Work out the finished part from the listing and answer in its coordinate system (mm). A direction names the side the tool comes from. Coordinates: 2 decimals unless noted, no trailing zeros. Order: outer loops, then holes, each group sorted by start corner. A loop starts at its lowest first (then second) coordinate and runs counter-clockwise, first axis right, second up. Notation, with made-up numbers: M 81,-30 L 137,-30 A17 cw 137,-20 Z; hole C -36.5,7 d2. An arc over 180 degrees is marked long. Use a Markdown table: item, result.
from build123d import *

# Parameters (mm, degrees)
SKETCH1_R           = 2.413
BOSS_EXTRUDE1_DEPTH = 45.212
SKETCH1_4_W         = 3.937
SKETCH1_4_H         = 2.794
BOSS_EXTRUDE2_DEPTH = 26.162
CUT_EXTRUDE1_START  = -24.892
SKETCH2_W           = 15.24
SKETCH2_H           = 11.43
SKETCH2_R           = 2.413
CUT_EXTRUDE1_DEPTH  = 24.892


with BuildPart() as part:
    # Sketch1 → Boss-Extrude1 (new body)
    with BuildSketch(Plane(origin=(0, 0, 0), x_dir=(1, 0, 0), z_dir=(0, 1, 0))):
        Polygon((40.25170153, 21.085507102), (40.25170153, 37.214507102), (21.20170153, 37.214507102), (21.20170153, 34.674507102), (8.50170153, 34.674507102), (8.50170153, 30.864507102), (21.20170153, 30.864507102), (21.20170153, 5.718507102), (8.50170153, 5.718507102), (8.50170153, 1.908507102), (21.20170153, 1.908507102), (21.20170153, -0.631492898), (40.25170153, -0.631492898), (40.25170153, 15.497507102), (32.37770153, 15.497507102), (32.37770153, 21.085507102), align=None)
        with Locations(Location((32.37770153, 5.591507102, 0), (0, 0, 90))):
            Circle(SKETCH1_R, mode=Mode.SUBTRACT)
        with Locations(Location((32.37770153, 30.991507102, 0), (0, 0, 90))):
            Circle(SKETCH1_R, mode=Mode.SUBTRACT)
    extrude(amount=BOSS_EXTRUDE1_DEPTH)

    # Sketch1_4 → Boss-Extrude2 (add)
    with BuildSketch(Plane(origin=(0, 0, 0), x_dir=(1, 0, 0), z_dir=(0, 1, 0))):
        with Locations((38.28320153, 19.688507102)):
            Rectangle(SKETCH1_4_W, SKETCH1_4_H)
        with Locations((34.34620153, 19.688507102)):
            Rectangle(SKETCH1_4_W, SKETCH1_4_H)
        with Locations((34.34620153, 16.894507102)):
            Rectangle(SKETCH1_4_W, SKETCH1_4_H)
        with Locations((38.28320153, 16.894507102)):
            Rectangle(SKETCH1_4_W, SKETCH1_4_H)
    extrude(amount=BOSS_EXTRUDE2_DEPTH)

    # Sketch2 → Cut-Extrude1 (cut)
    # profile 1 of 2: a face of its own
    with BuildSketch(Plane(origin=(0, 45.212, 0), x_dir=(1, 0, 0), z_dir=(0, 1, 0)).offset(CUT_EXTRUDE1_START)):
        with Locations((32.63170153, 5.083507102)):
            Rectangle(SKETCH2_W, SKETCH2_H)
        with Locations(Location((32.37770153, 5.591507102, 0), (0, 0, 90))):
            Circle(SKETCH2_R, mode=Mode.SUBTRACT)
    # profile 2 of 2: a face of its own
    with BuildSketch(Plane(origin=(0, 45.212, 0), x_dir=(1, 0, 0), z_dir=(0, 1, 0)).offset(CUT_EXTRUDE1_START)):
        with Locations((32.63170153, 31.499507102)):
            Rectangle(SKETCH2_W, SKETCH2_H)
        with Locations(Location((32.37770153, 30.991507102, 0), (0, 0, 90))):
            Circle(SKETCH2_R, mode=Mode.SUBTRACT)
    extrude(amount=CUT_EXTRUDE1_DEPTH, mode=Mode.SUBTRACT)


solid = part.part
(1) A cutting plane is placed at C-C (z = -30). Determine the outline of the cut face in (x, y).
Conclusion:
| item | result |
|---|---|
| outline | M 21.2,0 L 30.18,0 L 30.18,20.32 L 25.01,20.32 L 25.01,45.21 L 21.2,45.21 Z; M 34.58,0 L 40.25,0 L 40.25,20.32 L 34.58,20.32 Z |
(2) Straight lines are drawn through the part: L1, parallel to Z at x = 10, y = 12; L2, parallel to Z at x = 37, y = 28; L3, parallel to Z at x = 34.5, y = 14.5. For each, find the intervals that lie inside material, in ascending order.
Conclusion:
| item | result |
|---|---|
| L1 | -34.67 to -30.86, -5.72 to -1.91 |
| L2 | -25.78 to -21.09, -15.5 to -10.8 |
| L3 | -37.21 to -32.14, -29.84 to -6.74, -4.44 to 0.63 |
(3) A cutting plane is placed at B-B (y = 19). Determine the outline of the cut face in (x, z).
Conclusion:
| item | result |
|---|---|
| outline | M 8.5,-34.67 L 21.2,-34.67 L 21.2,-37.21 L 40.25,-37.21 L 40.25,0.63 L 21.2,0.63 L 21.2,-1.91 L 8.5,-1.91 L 8.5,-5.72 L 21.2,-5.72 L 21.2,-30.86 L 8.5,-30.86 Z; hole C 32.38,-30.99 d4.83; hole C 32.38,-5.59 d4.83 |
(4) Which of the six approach directions +Z, -Z, +X, -X, +Y, -Y give full straight-line access (tool end or side, diameter ignored) to faces 1 (the flat face through (34, 20.32, -33)), 2 (the flat face through (36, 36, -15.498)), 3 (the flat face through (21.202, 22, -1))?
Conclusion:
| item | result |
|---|---|
| face 1 | -Z, +X, +Y |
| face 2 | +X, +Y |
| face 3 | +Z, -X, +Y, -Y |
(5) A cutting plane is placed at A-A (x = 11). Determine the outline of the cut face in (y, z), then the cut area to 3 significant figures.
Conclusion:
| item | result |
|---|---|
| outline | M 0,-34.67 L 45.21,-34.67 L 45.21,-30.86 L 0,-30.86 Z; M 0,-5.72 L 45.21,-5.72 L 45.21,-1.91 L 0,-1.91 Z |
| area | 345 mm2 |
(6) Given P1, Ø5.5, axis at y = 29.5, z = -29, coming from the +X side; P2, Ø4, axis at x = 12, y = 17, coming from the +Z side; P3, Ø4, axis at x = 17.5, z = -9, coming from the -Y side; P4, Ø12, axis at x = 34, y = 36.5, coming from the -Z side, each flat-ended and moving along its own axis, determine where each tip first touches the part or whether it passes through.
Conclusion:
| item | result |
|---|---|
| P1 | x = 25.01 |
| P2 | z = -1.91 |
| P3 | through |
| P4 | z = -25.78 |
(7) A cutting plane is placed at D-D (x = 29). Determine the outline of the cut face in (y, z), then the cut area to 3 significant figures.
Conclusion:
| item | result |
|---|---|
| outline | M 0,-37.21 L 20.32,-37.21 L 20.32,-25.78 L 45.21,-25.78 L 45.21,-10.8 L 20.32,-10.8 L 20.32,0.63 L 0,0.63 Z |
| area | 1,140 mm2 |
(8) Determine the mould class of faces 4 (the flat face through (33, 33, -10.799)), 5 (the cylindrical face through (30.75, 10.02, -3.81)), 6 (the flat face through (25.012, 33, -31)) for opening direction X: pulls with the +X half, pulls with the -X half, needs draft (parallel to the pull), parting line crosses it, or undercut.
Conclusion:
| item | result |
|---|---|
| face 4 | needs draft |
| face 5 | undercut |
| face 6 | pulls with the +X half |
